Verification items for this drawing (mm, ordinates from the low corner). Give positions to 0.01 mm unless a question says otherwise; leave off trailing zeros. Loops run counter-clockwise (first coordinate to the right, second up) from the corner with the lowest first, then second, coordinate; pieces in that order, holes last. Notation, with made-up numbers: (18, 3) -> (68, 3) arc R26 ccw to (68, 24) -> close; hole circle Ø6 at (69, 42). An arc over 180 degrees is marked (long way). Answer in a Markdown table with one row per item. Add a question column.
Q1. Section check C-C on z = 13.5. Enter the section's corners in (x, y).
Q2. Section check A-A on y = 44.45. Enter the section's corners in (x, z).
Q3. Material ranges on probe 1 along Y at (x, z) = (50, 20); probe 2 along X at (y, z) = (43.5, 53); probe 3 along Y at (x, z) = (54.5, 47), recorded low to high.
Q4. Gauge pin test, flat ends, axial feed: P1, Ø5, axis at x = 70, z = 11.5, coming from the +Y side; P2, Ø8, axis at x = 36.5, z = 62.5, coming from the +Y side; P3, Ø6, axis at x = 51, z = 64.5, coming from the +Y side. Record the tip position at first contact, or that the pin passes through.
Q5. Section check D-D on x = 76.5. Enter the section's corners in (y, z).
Q6. Section check B-B on x = 50. Enter the section's corners in (y, z), and give its area (3 significant figures).
Q7. Release check for a two-part mould opening along Y. For the marked faces 1, 2 and 3 record: pulls with the +Y half, pulls with the -Y half, needs draft (parallel to the pull), parting line crosses it, or undercut.
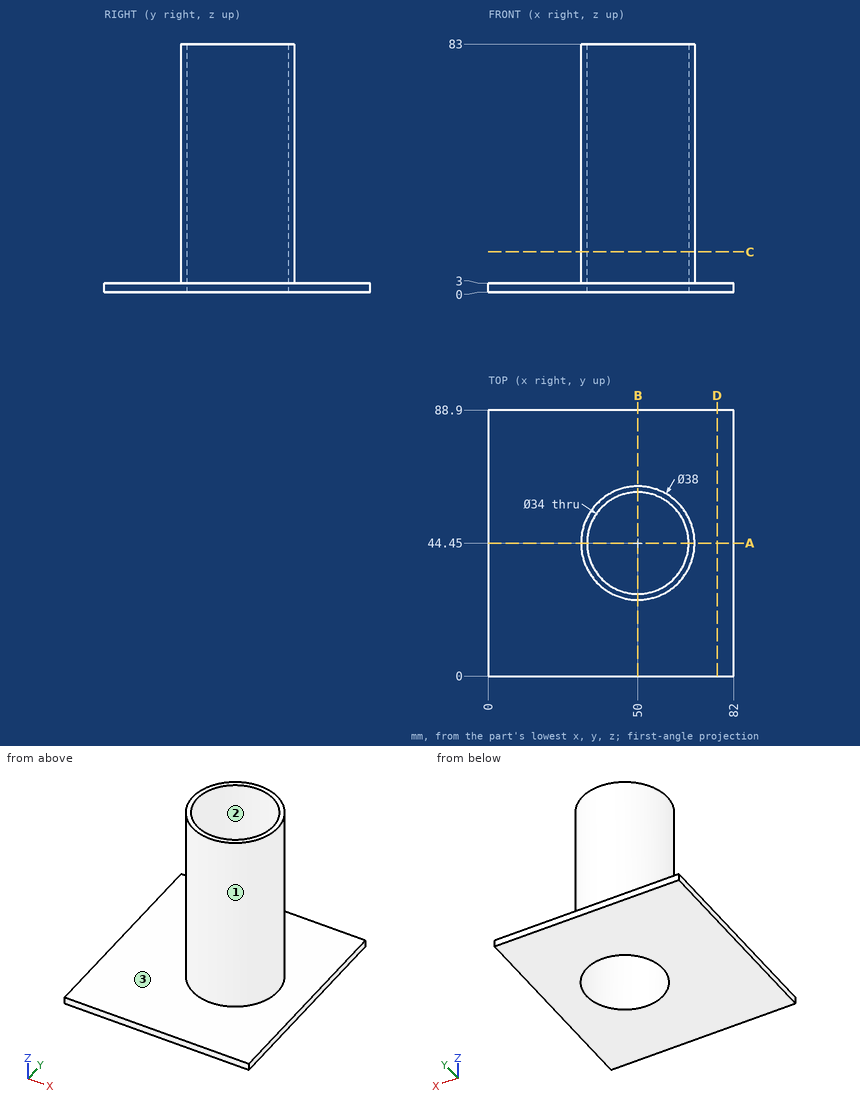
Taken from the geometry:
| question | item | result |
|---|---|---|
| 1 | outline | circle Ø38 at (50, 44.45); hole circle Ø34 at (50, 44.45) |
| 2 | outline | (0, 0) -> (33, 0) -> (33, 83) -> (31, 83) -> (31, 3) -> (0, 3) -> close; (67, 0) -> (82, 0) -> (82, 3) -> (69, 3) -> (69, 83) -> (67, 83) -> close |
| 3 | probe 1 | y = 25.45 to 27.45, 61.45 to 63.45 |
| 3 | probe 2 | x = 31.02 to 33.03, 66.97 to 68.98 |
| 3 | probe 3 | y = 25.99 to 28.06, 60.84 to 62.91 |
| 4 | P1 | stops at y = 51.85 |
| 4 | P2 | stops at y = 60.9 |
| 4 | P3 | stops at y = 63.45 |
| 5 | outline | (0, 0) -> (88.9, 0) -> (88.9, 3) -> (0, 3) -> close |
| 6 | outline | (0, 0) -> (27.45, 0) -> (27.45, 83) -> (25.45, 83) -> (25.45, 3) -> (0, 3) -> close; (61.45, 0) -> (88.9, 0) -> (88.9, 3) -> (63.45, 3) -> (63.45, 83) -> (61.45, 83) -> close |
| 6 | area | 485 mm² |
| 7 | face 1 | parting line crosses it |
| 7 | face 2 | undercut |
| 7 | face 3 | needs draft |
